Source: CAD feature listing. Evaluate the final solid. Frame: model axes, mm. A direction names the side the tool comes from. Round coordinates to 2 decimals unless told otherwise and drop trailing zeros. Loops run counter-clockwise (first coordinate to the right, second up) from the corner with the lowest first, then second, coordinate; pieces in that order, holes last. Notation, with made-up numbers: (88, 33.5) - (141, 33.5) arc R17 cw to (141, 61.5) - close; hole circle Ø1 at (-39.75, 4). An arc over 180 degrees is marked (long way). One line per question, with ' | ' between items.
from build123d import *

# Parameters (mm, degrees)
BOSS_EXTRUDE1_DEPTH = 14.1
BOSS_EXTRUDE2_DEPTH = 2
BOSS_EXTRUDE6_DEPTH = 21.5
SKETCH9_R           = 4.5
CUT_EXTRUDE6_DEPTH  = 20
SKETCH11_R          = 6
BOSS_EXTRUDE8_DEPTH = 2
CUT_EXTRUDE7_START  = 27
CUT_EXTRUDE7_DEPTH  = 27
SKETCH12_R          = 4.5
CUT_EXTRUDE8_DEPTH  = 12
SKETCH12_3_R        = 7.25
SKETCH12_3_R_2      = 5.5
CUT_EXTRUDE9_DEPTH  = 12
BOSS_EXTRUDE9_START = 7.1
SKETCH12_4_R        = 5.5
SKETCH12_4_R_2      = 4.5
BOSS_EXTRUDE9_DEPTH = 7.1
SKETCH13_W          = 0.8
SKETCH13_H          = 2.25
SKETCH13_W_2        = 0.7
SKETCH13_H_2        = 1.6
CUT_EXTRUDE10_DEPTH = 2
CUT_EXTRUDE12_DEPTH = 2


with BuildPart() as part:
    # Sketch1 → Boss-Extrude1 (new body)
    with BuildSketch(Plane.XY):
        with BuildLine():
            Line((8, -15.1), (8, 0))
            ThreePointArc((8, 0), (0, 8), (-8, 0))
            Line((-8, 0), (-8, -15.1))
            Line((-8, -15.1), (8, -15.1))
        make_face()
    extrude(amount=BOSS_EXTRUDE1_DEPTH)

    # Sketch2 → Boss-Extrude2 (add)
    with BuildSketch(Plane.XZ.offset(15.1)):
        with BuildLine():
            ThreePointArc((-7, 7.05), (-4.949747468, 2.100252532), (0, 0.05))
            Line((0, 0.05), (0, 7.05))
            Line((0, 7.05), (-7, 7.05))
        make_face()
        with BuildLine():
            Line((0, 7.05), (0, 0.05))
            ThreePointArc((0, 0.05), (4.949747468, 2.100252532), (7, 7.05))
            Line((7, 7.05), (0, 7.05))
        make_face()
        with BuildLine():
            Line((-7, 7.05), (0, 7.05))
            Line((0, 7.05), (0, 14.05))
            ThreePointArc((0, 14.05), (-4.949747468, 11.999747468), (-7, 7.05))
        make_face()
        with BuildLine():
            Line((0, 14.05), (0, 7.05))
            Line((0, 7.05), (7, 7.05))
            ThreePointArc((7, 7.05), (4.949747468, 11.999747468), (0, 14.05))
        make_face()
        with BuildLine():
            ThreePointArc((-7, 7.05), (-4.949747468, 2.100252532), (0, 0.05))
            Line((0, 0.05), (0, 7.05))
            Line((0, 7.05), (-7, 7.05))
        make_face()
        with BuildLine():
            Line((0, 7.05), (0, 0.05))
            ThreePointArc((0, 0.05), (4.949747468, 2.100252532), (7, 7.05))
            Line((7, 7.05), (0, 7.05))
        make_face()
        with BuildLine():
            Line((-7, 7.05), (0, 7.05))
            Line((0, 7.05), (0, 14.05))
            ThreePointArc((0, 14.05), (-4.949747468, 11.999747468), (-7, 7.05))
        make_face()
        with BuildLine():
            Line((0, 14.05), (0, 7.05))
            Line((0, 7.05), (7, 7.05))
            ThreePointArc((7, 7.05), (4.949747468, 11.999747468), (0, 14.05))
        make_face()
        with BuildLine():
            ThreePointArc((-7, 7.05), (-4.949747468, 2.100252532), (0, 0.05))
            Line((0, 0.05), (0, 7.05))
            Line((0, 7.05), (-7, 7.05))
        make_face()
        with BuildLine():
            Line((0, 7.05), (0, 0.05))
            ThreePointArc((0, 0.05), (4.949747468, 2.100252532), (7, 7.05))
            Line((7, 7.05), (0, 7.05))
        make_face()
        with BuildLine():
            Line((-7, 7.05), (0, 7.05))
            Line((0, 7.05), (0, 14.05))
            ThreePointArc((0, 14.05), (-4.949747468, 11.999747468), (-7, 7.05))
        make_face()
        with BuildLine():
            Line((0, 14.05), (0, 7.05))
            Line((0, 7.05), (7, 7.05))
            ThreePointArc((7, 7.05), (4.949747468, 11.999747468), (0, 14.05))
        make_face()
        with BuildLine():
            ThreePointArc((-7, 7.05), (-4.949747468, 2.100252532), (0, 0.05))
            Line((0, 0.05), (0, 7.05))
            Line((0, 7.05), (-7, 7.05))
        make_face()
        with BuildLine():
            Line((0, 7.05), (0, 0.05))
            ThreePointArc((0, 0.05), (4.949747468, 2.100252532), (7, 7.05))
            Line((7, 7.05), (0, 7.05))
        make_face()
        with BuildLine():
            Line((-7, 7.05), (0, 7.05))
            Line((0, 7.05), (0, 14.05))
            ThreePointArc((0, 14.05), (-4.949747468, 11.999747468), (-7, 7.05))
        make_face()
        with BuildLine():
            Line((0, 14.05), (0, 7.05))
            Line((0, 7.05), (7, 7.05))
            ThreePointArc((7, 7.05), (4.949747468, 11.999747468), (0, 14.05))
        make_face()
    extrude(amount=BOSS_EXTRUDE2_DEPTH)

    # Sketch8 → Boss-Extrude6 (add)
    with BuildSketch(Plane(origin=(0, -17.1, 0), x_dir=(-1, 0, 0), z_dir=(0, -1, 0))):
        with BuildLine():
            ThreePointArc((-4.949747468, -2.100252532), (-6.467156728, -4.371215973), (-7, -7.05))
            Line((-7, -7.05), (-4.949747468, -11.999747468))
            ThreePointArc((-4.949747468, -11.999747468), (-2.623124592, -13.539932001), (0.120272225, -14.04896668))
            Line((0.120272225, -14.04896668), (4.949747468, -11.999747468))
            ThreePointArc((4.949747468, -11.999747468), (6.467156728, -9.728784027), (7, -7.05))
            Line((7, -7.05), (4.949747468, -2.100252532))
            ThreePointArc((4.949747468, -2.100252532), (2.623124592, -0.560067999), (-0.120272225, -0.05103332))
            Line((-0.120272225, -0.05103332), (-4.949747468, -2.100252532))
        make_face()
    extrude(amount=BOSS_EXTRUDE6_DEPTH)

    # Sketch9 → Cut-Extrude6 (cut)
    with BuildSketch(Plane(origin=(0, -38.6, 0), x_dir=(-1, 0, 0), z_dir=(0, -1, 0))):
        with Locations(Location((0, -7.05, 0), (0, 0, 90))):
            Circle(SKETCH9_R)
    extrude(amount=-CUT_EXTRUDE6_DEPTH, mode=Mode.SUBTRACT)

    # Sketch11 → Boss-Extrude8 (add)
    with BuildSketch(Plane(origin=(0, -38.6, 0), x_dir=(-1, 0, 0), z_dir=(0, -1, 0))):
        with Locations(Location((0, -7.05, 0), (0, 0, 90))):
            Circle(SKETCH11_R)
    extrude(amount=BOSS_EXTRUDE8_DEPTH)

    # Sketch3 → Cut-Extrude7 (cut)
    with BuildSketch(Plane.XZ.offset(17.1).offset(CUT_EXTRUDE7_START)):
        with BuildLine():
            ThreePointArc((-4.5, 7.05), (-3.181980515, 3.868019485), (0, 2.55))
            Line((0, 2.55), (0, 7.05))
            Line((0, 7.05), (-4.5, 7.05))
        make_face()
        with BuildLine():
            Line((0, 7.05), (0, 2.55))
            ThreePointArc((0, 2.55), (3.181980515, 3.868019485), (4.5, 7.05))
            Line((4.5, 7.05), (0, 7.05))
        make_face()
        with BuildLine():
            Line((-4.5, 7.05), (0, 7.05))
            Line((0, 7.05), (0, 11.55))
            ThreePointArc((0, 11.55), (-3.181980515, 10.231980515), (-4.5, 7.05))
        make_face()
        with BuildLine():
            Line((0, 11.55), (0, 7.05))
            Line((0, 7.05), (4.5, 7.05))
            ThreePointArc((4.5, 7.05), (3.181980515, 10.231980515), (0, 11.55))
        make_face()
        with BuildLine():
            ThreePointArc((-4.5, 7.05), (-3.181980515, 3.868019485), (0, 2.55))
            Line((0, 2.55), (0, 7.05))
            Line((0, 7.05), (-4.5, 7.05))
        make_face()
        with BuildLine():
            Line((0, 7.05), (0, 2.55))
            ThreePointArc((0, 2.55), (3.181980515, 3.868019485), (4.5, 7.05))
            Line((4.5, 7.05), (0, 7.05))
        make_face()
        with BuildLine():
            Line((-4.5, 7.05), (0, 7.05))
            Line((0, 7.05), (0, 11.55))
            ThreePointArc((0, 11.55), (-3.181980515, 10.231980515), (-4.5, 7.05))
        make_face()
        with BuildLine():
            Line((0, 11.55), (0, 7.05))
            Line((0, 7.05), (4.5, 7.05))
            ThreePointArc((4.5, 7.05), (3.181980515, 10.231980515), (0, 11.55))
        make_face()
        with BuildLine():
            ThreePointArc((-4.5, 7.05), (-3.181980515, 3.868019485), (0, 2.55))
            Line((0, 2.55), (0, 7.05))
            Line((0, 7.05), (-4.5, 7.05))
        make_face()
        with BuildLine():
            Line((0, 7.05), (0, 2.55))
            ThreePointArc((0, 2.55), (3.181980515, 3.868019485), (4.5, 7.05))
            Line((4.5, 7.05), (0, 7.05))
        make_face()
        with BuildLine():
            Line((-4.5, 7.05), (0, 7.05))
            Line((0, 7.05), (0, 11.55))
            ThreePointArc((0, 11.55), (-3.181980515, 10.231980515), (-4.5, 7.05))
        make_face()
        with BuildLine():
            Line((0, 11.55), (0, 7.05))
            Line((0, 7.05), (4.5, 7.05))
            ThreePointArc((4.5, 7.05), (3.181980515, 10.231980515), (0, 11.55))
        make_face()
        with BuildLine():
            ThreePointArc((-4.5, 7.05), (-3.181980515, 3.868019485), (0, 2.55))
            Line((0, 2.55), (0, 7.05))
            Line((0, 7.05), (-4.5, 7.05))
        make_face()
        with BuildLine():
            Line((0, 7.05), (0, 2.55))
            ThreePointArc((0, 2.55), (3.181980515, 3.868019485), (4.5, 7.05))
            Line((4.5, 7.05), (0, 7.05))
        make_face()
        with BuildLine():
            Line((-4.5, 7.05), (0, 7.05))
            Line((0, 7.05), (0, 11.55))
            ThreePointArc((0, 11.55), (-3.181980515, 10.231980515), (-4.5, 7.05))
        make_face()
        with BuildLine():
            Line((0, 11.55), (0, 7.05))
            Line((0, 7.05), (4.5, 7.05))
            ThreePointArc((4.5, 7.05), (3.181980515, 10.231980515), (0, 11.55))
        make_face()
    extrude(amount=-CUT_EXTRUDE7_DEPTH, mode=Mode.SUBTRACT)

    # Sketch12 → Cut-Extrude8 (cut)
    with BuildSketch(Plane.XY.offset(14.1)):
        Circle(SKETCH12_R)
    extrude(amount=-CUT_EXTRUDE8_DEPTH, mode=Mode.SUBTRACT)

    # Sketch12_3 → Cut-Extrude9 (cut)
    with BuildSketch(Plane.XY.offset(14.1)):
        Circle(SKETCH12_3_R)
        Circle(SKETCH12_3_R_2, mode=Mode.SUBTRACT)
    extrude(amount=-CUT_EXTRUDE9_DEPTH, mode=Mode.SUBTRACT)

    # Sketch12_4 → Boss-Extrude9 (add)
    with BuildSketch(Plane.XY.offset(14.1).offset(BOSS_EXTRUDE9_START)):
        Circle(SKETCH12_4_R)
        Circle(SKETCH12_4_R_2, mode=Mode.SUBTRACT)
    extrude(amount=-BOSS_EXTRUDE9_DEPTH)

    # Sketch13 → Cut-Extrude10 (cut)
    with BuildSketch(Plane.ZY.offset(8)):
        with Locations((10.5, -7.641192761)):
            Rectangle(SKETCH13_W, SKETCH13_H)
        with Locations((11.8, -10.441164669)):
            Rectangle(SKETCH13_W_2, SKETCH13_H_2)
        with Locations((9.2, -10.441164669)):
            Rectangle(SKETCH13_W_2, SKETCH13_H_2)
    extrude(amount=-CUT_EXTRUDE10_DEPTH, mode=Mode.SUBTRACT)

    # Sketch14 → Cut-Extrude12 (cut)
    with BuildSketch(Plane(origin=(8, 0, 0), x_dir=(0, 0, -1), z_dir=(1, 0, 0))):
        with BuildLine():
            Line((-7.64754844, -14.165884792), (-11.64754844, -14.165884792))
            ThreePointArc((-11.64754844, -14.165884792), (-12.354655221, -13.872991573), (-12.64754844, -13.165884792))
            Line((-12.64754844, -13.165884792), (-12.64754844, -7.165884792))
            ThreePointArc((-12.64754844, -7.165884792), (-12.354655221, -6.45877801), (-11.64754844, -6.165884792))
            Line((-11.64754844, -6.165884792), (-7.64754844, -6.165884792))
            ThreePointArc((-7.64754844, -6.165884792), (-6.940441659, -6.45877801), (-6.64754844, -7.165884792))
            Line((-6.64754844, -7.165884792), (-6.64754844, -13.165884792))
            ThreePointArc((-6.64754844, -13.165884792), (-6.940441659, -13.872991573), (-7.64754844, -14.165884792))
        make_face()
        with BuildLine():
            Line((-9.441476419, -12.684690809), (-9.85362046, -12.684690809))
            ThreePointArc((-9.85362046, -12.684690809), (-10.914280632, -12.245350981), (-11.35362046, -11.184690809))
            Line((-11.35362046, -11.184690809), (-11.35362046, -9.147078774))
            ThreePointArc((-11.35362046, -9.147078774), (-10.914280632, -8.086418602), (-9.85362046, -7.647078774))
            Line((-9.85362046, -7.647078774), (-9.441476419, -7.647078774))
            ThreePointArc((-9.441476419, -7.647078774), (-8.380816248, -8.086418602), (-7.941476419, -9.147078774))
            Line((-7.941476419, -9.147078774), (-7.941476419, -11.184690809))
            ThreePointArc((-7.941476419, -11.184690809), (-8.380816248, -12.245350981), (-9.441476419, -12.684690809))
        make_face(mode=Mode.SUBTRACT)
    extrude(amount=-CUT_EXTRUDE12_DEPTH, mode=Mode.SUBTRACT)


solid = part.part
1. Access query for faces 1 (the flat face through (-7, -10, 12.15)), 2 (the flat face through (0, -17.1, 7)), 3 (the cylindrical face through (7.014, -6.467, 12.362)). Directions: +Z, -Z, +X, -X, +Y, -Y. A direction counts if a zero-diameter tool reaches every point of the face in a straight line with its end or side. Return the directions, or none.
Worked out:
face 1: -X | face 2: -Y | face 3: +X
2. Contact query for flat-ended pins moving along their axis: P1, Ø1, axis at x = -2.5, z = 13.5, coming from the -Y side; P2, Ø7, axis at x = 0, y = -0.5, coming from the +Z side; P3, Ø4, axis at x = 2.5, z = 17, coming from the -Y side; P4, Ø0.6, axis at x = 7.5, y = -10, coming from the -Z side. Output: stop coordinate, or through.
Worked out:
P1: stops at y = -38.6 | P2: stops at z = 2.1 | P3: stops at y = -5.48 | P4: stops at z = 0
3. Section query A-A, the plane z = 3.5. Return loops of the section in (x, y), plus the area to 3 significant figures.
Worked out:
outline: (-8, -15.1) - (-6.03, -15.1) - (-6.03, -17.1) - (-5.53, -17.1) - (-5.53, -38.6) - (-4.84, -38.6) - (-4.84, -40.6) - (-2.77, -40.6) - (-2.77, -17.1) - (2.77, -17.1) - (2.77, -40.6) - (4.84, -40.6) - (4.84, -38.6) - (6.03, -38.6) - (6.03, -15.1) - (8, -15.1) - (8, 0) arc R8 ccw to (-8, 0) - close; circle Ø11 at (0, 0); hole circle Ø14.5 at (0, 0); hole circle Ø9 at (0, 0) | area: 371 mm2
4. Mould query, pull axis Y, two halves, no side actions, for faces 4 (the flat face through (-7, -8, 10.1)), 5 (the flat face through (-2, -38.6, 1)), 6 (the flat face through (-5, 0, 21.2)). Classes: released by +Y, released by -Y, zero draft, split by the parting line, or undercut.
Worked out:
face 4: undercut | face 5: released by -Y | face 6: zero draft
5. Section query C-C, the plane z = 16. Return loops of the section in (x, y).
Worked out:
outline: circle Ø11 at (0, 0); hole circle Ø9 at (0, 0)
6. Material intervals for probe 1 along Y at (x, z) = (0, 10.25); probe 2 along X at (y, z) = (-29.5, 7.05); probe 3 along Y at (x, z) = (-1.25, 2.25), sorted ascending.
Worked out:
probe 1: y = -17.1 to -7.25, -5.5 to -4.5, 4.5 to 5.5, 7.25 to 8 | probe 2: x = -7 to -4.5, 4.5 to 7 | probe 3: y = -40.6 to -7.14, -5.36 to -4.32, 4.32 to 5.36, 7.14 to 7.9
